Verification items for the finished model (mm, model axes). A direction names the side the tool comes from. Round coordinates to 2 decimals unless told otherwise and drop trailing zeros. Write each loop counter-clockwise with the first axis right and the second up, starting at its lowest first coordinate (ties: lowest second). Pieces come first, ordered by that corner, then holes. Notation, with made-up numbers: (59.25, 67) - (111.25, 67) arc R17 ccw to (111.25, 75) - close; hole circle Ø5 at (79.5, -0.75). An arc over 180 degrees is marked (long way). Answer as a JSON object with one key per item and string values. Group by question number.
1) Section check A-A (x = 0). Enter the section's corners in (y, z) (3 decimals).
2) Go/stop test with flat-tipped pins: pin 1 Ø1.6 at (y, z) = (10.5, -2) entering from +X; pin 2 Ø1 at (x, z) = (19, -1.5) entering from +Y (3 decimals); pin 3 Ø6 at (x, z) = (12.5, -11.96) entering from +Y. Record where each tip stops, or that it passes through.
3) Section check D-D (x = 12.5). Enter the section's corners in (y, z) (3 decimals), then the cut area to 3 significant figures.
4) Set-up check for faces 1 (the flat face through (-12, 9, -2)), 2 (the flat face through (0, -2, -20)), 3 (the flat face through (0, 5, -3.175)), 4 (the flat face through (19, 3.175, -2)): record each of +Z, -Z, +X, -X, +Y, -Y from which the full face is reachable in a straight line by a thin tool's end or side.
5) Section check C-C (z = -8.5). Enter the section's corners in (x, y) (3 decimals).
6) Section check B-B (y = 8.25). Enter the section's corners in (x, z) (3 decimals), then the cut area to 3 significant figures.
7) Thickness scan on line 1 (Z direction, x = 9, y = 6) (3 decimals); line 2 (Y direction, x = 0, z = -1.1) (3 decimals). Record the ranges inside material, lowest first.
8) Mould release check, pull along X, two halves, no side actions. Record for faces 5 (the cylindrical face through (-10.66, -1.61, -13.65)), 6 (the flat face through (0, 5, 0)), 7 (the cylindrical face through (14.34, -1.61, -13.65)), 8 (the cylindrical face through (-24.4, -1.57, -19.43)): +X half, -X half, draft (parallel to the pull), parting line (faces both ways), or undercut.
```python
from build123d import *

# Parameters (mm, degrees)
SKETCH1_R                    = 6.5
BASE_FLANGE1_DEPTH           = 3.175
EDGE_FLANGE1_STRIP_W         = 14.1732
EDGE_FLANGE1_STRIP_H         = 3.175
EDGE_FLANGE1_STRIP_CUT_DEPTH = 50
EDGE_FLANGE1_DEPTH           = 50
FILLET2_R                    = 2
F_5_0MM_DOWEL_HOLE1_D        = 5


# Sheet-metal steps are written as plain solids
with BuildPart() as part:
    # Sketch1 → Base-Flange1 (new body)
    with BuildSketch(Plane.XY):
        with BuildLine():
            Line((-25, 0), (25, 0))
            Line((25, 0), (25, 1.175))
            ThreePointArc((25, 1.175), (24.414213562, 2.589213562), (23, 3.175))
            Line((23, 3.175), (14, 3.175))
            ThreePointArc((14, 3.175), (12.585786438, 3.760786438), (12, 5.175))
            Line((12, 5.175), (12, 13.175))
            ThreePointArc((12, 13.175), (0, 25.175), (-12, 13.175))
            Line((-12, 13.175), (-12, 5.175))
            ThreePointArc((-12, 5.175), (-12.585786438, 3.760786438), (-14, 3.175))
            Line((-14, 3.175), (-23, 3.175))
            ThreePointArc((-23, 3.175), (-24.414213562, 2.589213562), (-25, 1.175))
            Line((-25, 1.175), (-25, 0))
        make_face()
        with Locations((0, 13.175)):
            Circle(SKETCH1_R, mode=Mode.SUBTRACT)
    extrude(amount=-BASE_FLANGE1_DEPTH)

    # Edge-Flange1 strip (across the edge) → Edge-Flange1 strip cut (cut)
    with BuildSketch(Plane(origin=(25, 0, -3.175), x_dir=(0, 1, 0), z_dir=(-1, 0, 0))):
        with Locations((-6.35, -1.5875)):
            Rectangle(EDGE_FLANGE1_STRIP_W, EDGE_FLANGE1_STRIP_H)
    extrude(amount=EDGE_FLANGE1_STRIP_CUT_DEPTH, mode=Mode.SUBTRACT)

    # Edge-Flange1 section (across the edge) → Edge-Flange1 (add)
    with BuildSketch(Plane(origin=(25, 0, -3.175), x_dir=(0, 1, 0), z_dir=(-1, 0, 0))):
        with BuildLine():
            Line((-3.175, 0.7366), (-3.175, 16.825))
            Line((-3.175, 16.825), (0, 16.825))
            Line((0, 16.825), (0, 0.7366))
            ThreePointArc((0, 0.7366), (0.215745145, 0.215745145), (0.7366, 0))
            Line((0.7366, 0), (0.7366, -3.175))
            ThreePointArc((0.7366, -3.175), (-2.029318885, -2.029318885), (-3.175, 0.7366))
        make_face()
    extrude(amount=EDGE_FLANGE1_DEPTH)

    # Fillet2
    fillet2_edges = [part.edges().sort_by_distance(p)[0] for p in [
        (25, -1.5875, -20),
        (-25, -1.5875, -20),
    ]]
    fillet(fillet2_edges, radius=FILLET2_R)

    # Ø5.0mm Dowel Hole1 (through all)
    with Locations(Plane(origin=(0, 0, 0), x_dir=(1, 0, 0), z_dir=(0, 1, 0))):
        with Locations((-12.5, 11.9558), (12.5, 11.9558)):
            Hole(F_5_0MM_DOWEL_HOLE1_D / 2)


solid = part.part
```
Returned:
{
 "1": {"outline": "(-3.175, -20) - (0, -20) - (0, -3.912) arc R0.737 cw to (0.737, -3.175) - (6.675, -3.175) - (6.675, 0) - (0.737, 0) arc R3.912 ccw to (-3.175, -3.912) - close; (19.675, -3.175) - (25.175, -3.175) - (25.175, 0) - (19.675, 0) - close"},
 "2": {"pin 1": "x = 12", "pin 2": "y = 3.175", "pin 3": "y = 0"},
 "3": {"outline": "(-3.175, -20) - (0, -20) - (0, -14.456) - (-3.175, -14.456) - close; (-3.175, -9.456) - (0, -9.456) - (0, -3.912) arc R0.737 cw to (0.737, -3.175) - (3.852, -3.175) - (3.852, 0) - (0.737, 0) arc R3.912 ccw to (-3.175, -3.912) - close", "area": "56.7 mm2"},
 "4": {"face 1": "+Z, -Z, -X, +Y", "face 2": "-Z, +X, -X, +Y, -Y", "face 3": "-Z, +X, -X, +Y", "face 4": "+Z, -Z, +X, +Y"},
 "5": {"outline": "(-25, -3.175) - (25, -3.175) - (25, 0) - (-25, 0) - close"},
 "6": {"outline": "(-12, -3.175) - (-4.242, -3.175) - (-4.242, 0) - (-12, 0) - close; (4.242, -3.175) - (12, -3.175) - (12, 0) - (4.242, 0) - close", "area": "49.3 mm2"},
 "7": {"line 1": "-3.175 to 0", "line 2": "-1.983 to 6.675, 19.675 to 25.175"},
 "8": {"face 5": "undercut", "face 6": "draft", "face 7": "undercut", "face 8": "-X half"}
}
